Study the drawing (mm; zero at the part's minimum x, y, z) and answer. Coordinates: 2 decimals unless noted, no trailing zeros. Write each loop counter-clockwise with the first axis right and the second up, starting at its lowest first coordinate (ties: lowest second). Pieces come first, ordered by that corner, then holes. Notation, with made-up numbers: (33.25, 66) -> (37.25, 66) arc R14 ccw to (37.25, 76) -> close; hole circle Ø2 at (-34, -19). An arc over 180 degrees is marked (long way). Answer in a Markdown table with one row per item. Add a question column.
Item 1: Straight lines are drawn through the part: line 1 (X direction, y = 3.65, z = 5.5); line 2 (Z direction, x = 38, y = 2.4); line 3 (X direction, y = 1.5, z = 35). For each, find the intervals that lie inside material, in ascending order. Write a range as from..to.
Item 2: Section C-C on x = 55 is taken. Write down the section's boundary in (y, z), then the cut area to 3 significant figures.
Item 3: Section A-A on z = 85.5 is taken. Write down the section's boundary in (x, y), then the cut area to 3 significant figures.
Item 4: Section B-B on y = 3.85 is taken. Write down the section's boundary in (x, z).
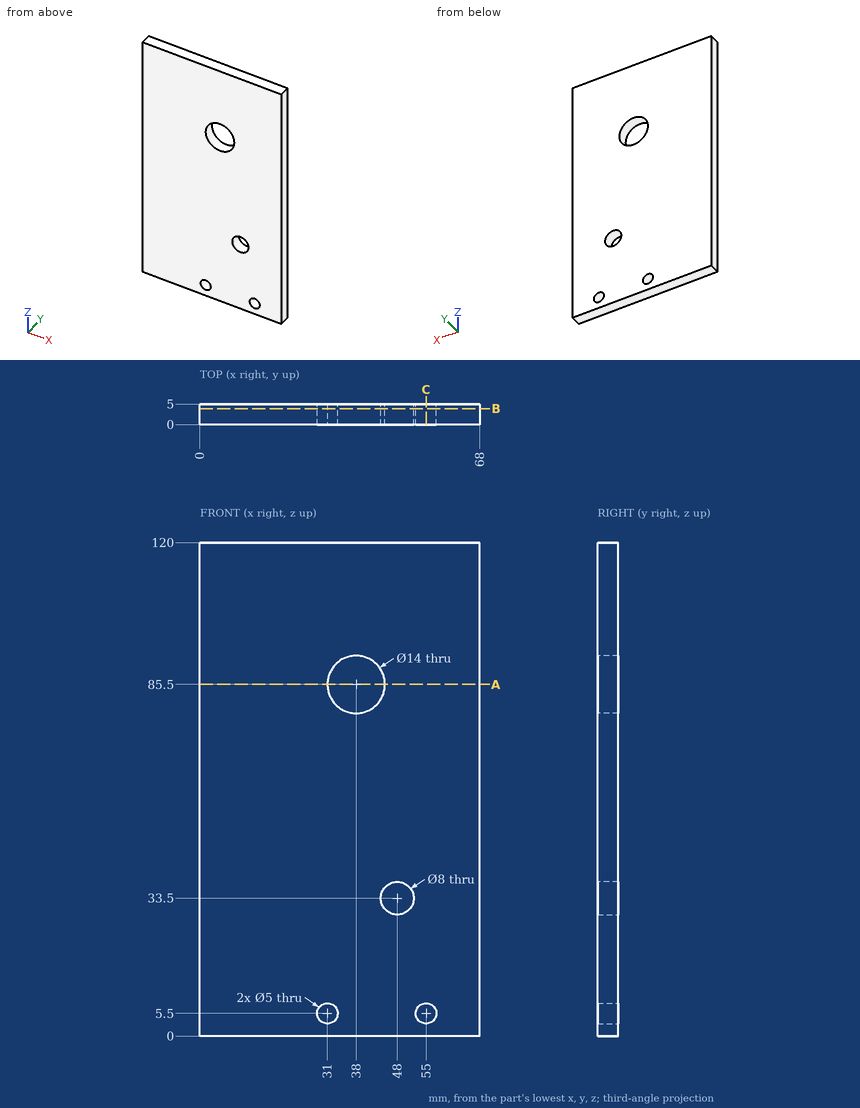
Results below:
| question | item | result |
|---|---|---|
| 1 | line 1 | x = 0..28.5, 33.5..52.5, 57.5..68 |
| 1 | line 2 | z = 0..78.5, 92.5..120 |
| 1 | line 3 | x = 0..44.29, 51.71..68 |
| 2 | outline | (0, 0) -> (5, 0) -> (5, 3) -> (0, 3) -> close; (0, 8) -> (5, 8) -> (5, 120) -> (0, 120) -> close |
| 2 | area | 575 mm2 |
| 3 | outline | (0, 0) -> (31, 0) -> (31, 5) -> (0, 5) -> close; (45, 0) -> (68, 0) -> (68, 5) -> (45, 5) -> close |
| 3 | area | 270 mm2 |
| 4 | outline | (0, 0) -> (68, 0) -> (68, 120) -> (0, 120) -> close; hole circle Ø5 at (31, 5.5); hole circle Ø14 at (38, 85.5); hole circle Ø8 at (48, 33.5); hole circle Ø5 at (55, 5.5) |
